Could you check a few things on this drawing? It's one solid part, dimensions in mm from its lowest x, y, z. Give positions to 0.01 mm unless a question says otherwise; leave off trailing zeros. Loops run counter-clockwise (first coordinate to the right, second up) from the corner with the lowest first, then second, coordinate; pieces in that order, holes last.
1. Imagine slicing it at C-C (y = 0.55). Count the separate pieces of the cut face and the enclosed holes in it, plus the area to 3 significant figures.
2. I need wall thicknesses on line 1 along Z through (x, y) = (12.7, 0.6) (1 decimal); line 2 along Z through (x, y) = (20, 0.35); line 3 along Z through (x, y) = (19.5, 0.2) (1 decimal). Which ranges of each line are inside material? Lowest first, please.
3. Imagine slicing it at A-A (z = 82.55). List the corners of the cut face in (x, y) for me.
4. Imagine slicing it at B-B (x = 12.7). List the corners of the cut face in (y, z) for me (1 decimal).
5. Imagine slicing it at D-D (z = 36). List the corners of the cut face in (x, y) for me.
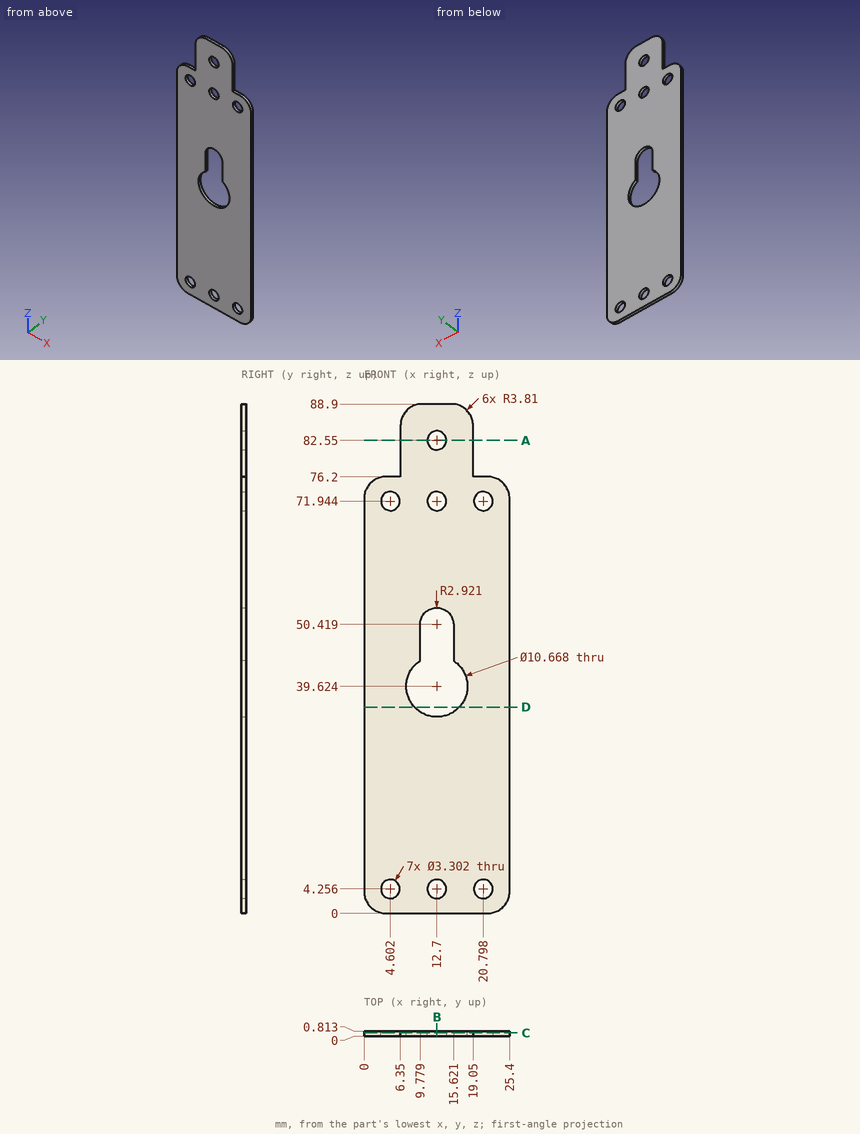
Derived:
1. separate pieces: 1
1. enclosed holes: 8
1. area: 1,880 mm2
2. line 1: z = 0 to 2.6, 5.9 to 34.3, 53.3 to 70.3, 73.6 to 80.9, 84.2 to 88.9
2. line 2: z = 0 to 2.81, 5.7 to 70.5, 73.39 to 76.2
2. line 3: z = 0 to 3.2, 5.3 to 70.9, 73 to 76.2
3. outline: (6.35, 0) - (11.05, 0) - (11.05, 0.81) - (6.35, 0.81) - close; (14.35, 0) - (19.05, 0) - (19.05, 0.81) - (14.35, 0.81) - close
4. outline: (0, 0) - (0.8, 0) - (0.8, 2.6) - (0, 2.6) - close; (0, 5.9) - (0.8, 5.9) - (0.8, 34.3) - (0, 34.3) - close; (0, 53.3) - (0.8, 53.3) - (0.8, 70.3) - (0, 70.3) - close; (0, 73.6) - (0.8, 73.6) - (0.8, 80.9) - (0, 80.9) - close; (0, 84.2) - (0.8, 84.2) - (0.8, 88.9) - (0, 88.9) - close
5. outline: (0, 0) - (8.79, 0) - (8.79, 0.81) - (0, 0.81) - close; (16.61, 0) - (25.4, 0) - (25.4, 0.81) - (16.61, 0.81) - close
